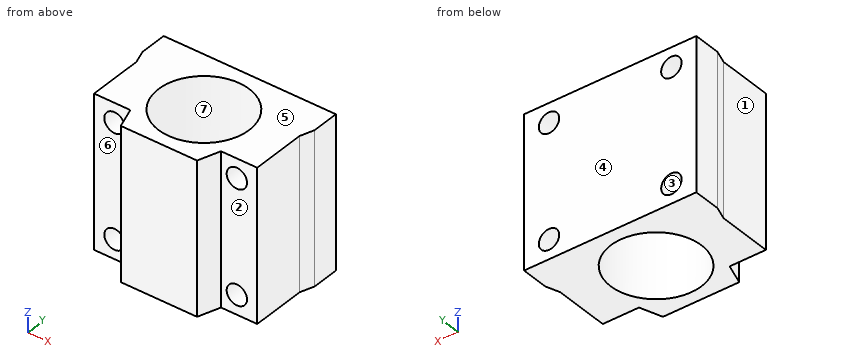
from build123d import *

# Parameters (mm, degrees)
DODANIE_WYCI_GNI_CIE1_DEPTH      = 33.5
DODANIE_WYCI_GNI_CIE1_DEPTH_BACK = 33.5
SZKIC1_R                         = 20
OTW_R_POD_RUB_M81_D              = 9
LUSTRO2_COPY_1_D                 = 9


with BuildPart() as part:
    # Szkic1 → Dodanie-wyciągnięcie1 (new, two sides: drawn at the far end of the back side and taken through both)
    with BuildSketch(Plane.XY.offset(-DODANIE_WYCI_GNI_CIE1_DEPTH_BACK)):
        Polygon((16.833333333, -25.5), (-16.833333333, -25.5), (-20, -16), (-36, -16), (-36, 8), (-38, 14), (-38, 26), (38, 26), (38, 14), (36, 8), (36, -16), (20, -16), align=None)
        Circle(SZKIC1_R, mode=Mode.SUBTRACT)
    extrude(amount=DODANIE_WYCI_GNI_CIE1_DEPTH + DODANIE_WYCI_GNI_CIE1_DEPTH_BACK)

    # Otwór pod śrubę M81 (through all)
    with Locations(Plane(origin=(0, -16, 0), x_dir=(-1, 0, 0), z_dir=(0, -1, 0))):
        with Locations((-27, -25)):
            otw_r_pod_rub_m81 = Hole(OTW_R_POD_RUB_M81_D / 2)

    # Lustro1: Otwór pod śrubę M81 across plane
    add(otw_r_pod_rub_m81.mirror(Plane(origin=(0, 0, 0), x_dir=(0, 0, 1), z_dir=(1, 0, 0))), mode=Mode.SUBTRACT)

    # Lustro2: Otwór pod śrubę M81 across plane
    add(otw_r_pod_rub_m81.mirror(Plane.XY), mode=Mode.SUBTRACT)

    # Lustro2 copy 1 (through all)
    with Locations(Plane.XZ.offset(16)):
        with Locations((-27, -25)):
            Hole(LUSTRO2_COPY_1_D / 2)


solid = part.part
Work out the finished part from the listing and answer in its coordinate system (mm). Face numbers are marked on the shaded views. A direction names the side the tool comes from. Coordinates: 2 decimals unless noted, no trailing zeros. Order: outer loops, then holes, each group sorted by start corner. A loop starts at its lowest first (then second) coordinate and runs counter-clockwise, first axis right, second up. Notation, with made-up numbers: (32, 29.5) - (42, 29.5) arc R27 cw to (42, 55.5) - close; hole circle Ø4 at (-1.5, -34.5). An arc over 180 degrees is marked (long way). Put each result on its own line as item: value. Start each with the question number.
1) For the marked faces 1, 2 and 3, determine the directions among +Z, -Z, +X, -X, +Y, -Y from which every point of the face is accessible in a straight line to the end or side of a thin tool.
2) Find the intervals of material crossed by line 1 (Z direction, x = 27, y = 4); line 2 (Z direction, x = -23.5, y = -13.5); line 3 (X direction, y = 0.5, z = -23), in increasing order. Write a range as from..to.
3) Find section D-D (x = 0). Give the vertices of the cut face in (y, z), plus the area to 4 significant figures.
4) Find section A-A (z = 25). Give the vertices of the cut face in (x, y).
5) For a pull along Y with two mould halves and no side action, classify the marked faces 4, 5, 6 and 7 as released by +Y, released by -Y, zero draft, split by the parting line, or undercut.
6) Flat-ended cylindrical pins translate along their axes: pin 1 (6 mm diameter, centred on x = -13, y = -9.5, fed in from -Z); pin 2 (12 mm diameter, centred on y = -13, z = -22.5, fed in from -X); pin 3 (2 mm diameter, centred on y = -2.5, z = 7.5, fed in from +X); pin 4 (2 mm diameter, centred on x = -29, z = -14, fed in from -Y). Find the tip coordinate at first contact, or state that the pin passes through.
7) Find section B-B (y = 0). Give the vertices of the cut face in (x, z).
8) Find section C-C (x = 27). Give the vertices of the cut face in (y, z).
Results list:
1. face 1: +Z, -Z, -X, -Y
1. face 2: +Z, -Z, +X, -Y
1. face 3: +Y, -Y
2. line 1: z = -33.5..-29.5, -20.5..20.5, 29.5..33.5
2. line 2: z = -33.5..-27.83, -22.17..22.17, 27.83..33.5
2. line 3: x = -36..-31.03, -22.97..-19.99, 19.99..22.97, 31.03..36
3. outline: (-25.5, -33.5) - (-20, -33.5) - (-20, 33.5) - (-25.5, 33.5) - close; (20, -33.5) - (26, -33.5) - (26, 33.5) - (20, 33.5) - close
3. area: 770.5 mm^2
4. outline: (-38, 14) - (-36, 8) - (-36, -16) - (-31.5, -16) - (-31.5, 26) - (-38, 26) - close; (-22.5, -16) - (-20, -16) - (-16.83, -25.5) - (16.83, -25.5) - (20, -16) - (22.5, -16) - (22.5, 26) - (-22.5, 26) - close; (31.5, -16) - (36, -16) - (36, 8) - (38, 14) - (38, 26) - (31.5, 26) - close; hole circle Ø40 at (0, 0)
5. face 4: released by +Y
5. face 5: zero draft
5. face 6: released by -Y
5. face 7: undercut
6. pin 1: passes through
6. pin 2: stops at x = -36
6. pin 3: stops at x = 36
6. pin 4: stops at y = -16
7. outline: (-36, -33.5) - (-20, -33.5) - (-20, 33.5) - (-36, 33.5) - close; (20, -33.5) - (36, -33.5) - (36, 33.5) - (20, 33.5) - close; hole circle Ø9 at (-27, -25); hole circle Ø9 at (-27, 25); hole circle Ø9 at (27, -25); hole circle Ø9 at (27, 25)
8. outline: (-16, -33.5) - (26, -33.5) - (26, -29.5) - (-16, -29.5) - close; (-16, -20.5) - (26, -20.5) - (26, 20.5) - (-16, 20.5) - close; (-16, 29.5) - (26, 29.5) - (26, 33.5) - (-16, 33.5) - close
